```python
from build123d import *

# Parameters (mm, degrees)
SKETCH1_W           = 200
SKETCH1_H           = 35
BOSS_EXTRUDE1_DEPTH = 3
FILLET1_R           = 15
CUT_EXTRUDE1_DEPTH  = 102.564019219


with BuildPart() as part:
    # Sketch1 → Boss-Extrude1 (new body)
    with BuildSketch(Plane(origin=(0, 0, 0), x_dir=(1, 0, 0), z_dir=(0, 1, 0))):
        Rectangle(SKETCH1_W, SKETCH1_H)
    extrude(amount=BOSS_EXTRUDE1_DEPTH)

    # Fillet1
    fillet1_edges = [part.edges().sort_by_distance(p)[0] for p in [
        (100, 1.5, -17.5),
        (100, 1.5, 17.5),
    ]]
    fillet(fillet1_edges, radius=FILLET1_R)

    # Sketch2 → Cut-Extrude1 (cut, through all)
    with BuildSketch(Plane(origin=(0, 3, 0), x_dir=(1, 0, 0), z_dir=(0, 1, 0))):
        with BuildLine():
            ThreePointArc((-93.377001476, 15), (-96.147633262, 16.147633262), (-95, 13.377001476))
            Line((-95, 13.377001476), (-95, 15))
            Line((-95, 15), (-93.377001476, 15))
        make_face()
        with BuildLine():
            Line((-95, 15), (-95, 13.377001476))
            ThreePointArc((-95, 13.377001476), (-93.852366738, 13.852366738), (-93.377001476, 15))
            Line((-93.377001476, 15), (-95, 15))
        make_face()
        with BuildLine():
            ThreePointArc((-95, -13.5), (-96.060660172, -16.060660172), (-93.5, -15))
            Line((-93.5, -15), (-95, -15))
            Line((-95, -15), (-95, -13.5))
        make_face()
        with BuildLine():
            Line((-95, -15), (-93.5, -15))
            ThreePointArc((-93.5, -15), (-93.939339828, -13.939339828), (-95, -13.5))
            Line((-95, -13.5), (-95, -15))
        make_face()
        with BuildLine():
            ThreePointArc((-63.143993753, -13.5), (-64.204653925, -13.939339828), (-64.643993753, -15))
            Line((-64.643993753, -15), (-63.143993753, -15))
            Line((-63.143993753, -15), (-63.143993753, -13.5))
        make_face()
        with BuildLine():
            Line((-63.143993753, -15), (-64.643993753, -15))
            ThreePointArc((-64.643993753, -15), (-63.143993753, -16.5), (-61.643993753, -15))
            ThreePointArc((-61.643993753, -15), (-62.083333581, -13.939339828), (-63.143993753, -13.5))
            Line((-63.143993753, -13.5), (-63.143993753, -15))
        make_face()
        with BuildLine():
            ThreePointArc((-64.643993753, 15), (-64.204653925, 13.939339828), (-63.143993753, 13.5))
            Line((-63.143993753, 13.5), (-63.143993753, 15))
            Line((-63.143993753, 15), (-64.643993753, 15))
        make_face()
        with BuildLine():
            Line((-63.143993753, 15), (-63.143993753, 13.5))
            ThreePointArc((-63.143993753, 13.5), (-62.083333581, 13.939339828), (-61.643993753, 15))
            ThreePointArc((-61.643993753, 15), (-63.143993753, 16.5), (-64.643993753, 15))
            Line((-64.643993753, 15), (-63.143993753, 15))
        make_face()
    extrude(amount=-CUT_EXTRUDE1_DEPTH, mode=Mode.SUBTRACT)


solid = part.part
```
CAD build for the part. Positions are in the model's coordinates, mm. Give positions to 0.01 mm unless a question says otherwise; leave off trailing zeros. Write each loop counter-clockwise with the first axis right and the second up, starting at its lowest first coordinate (ties: lowest second). Pieces come first, ordered by that corner, then holes. Notation, with made-up numbers: M -25,-34 L -3,-34 A18 cw -3,-2 Z; hole C 41,-32 d10. An arc over 180 degrees is marked long. Return JSON: item names as keys, results as strings. Group by question number.
(1) Band-saw the part on A-A (y = 2.45). Give the cut face in (x, z), and give its area (3 significant figures).
(2) Drill centre lines: L1, parallel to Z at x = -95, y = 2.2; L2, parallel to X at y = 1.5, z = -15; L3, parallel to X at y = 2, z = 15. Where is each one in solid material? Low to high. Write a range as [from, to].
(3) Flat gauge pin, fed straight in: pin 1 Ø2.5 at (x, z) = (-95, -15) entering from -Y. Where does the tip first touch, or does it go through?
Entries:
{
 "1": {"outline": "M -100,-17.5 L 85,-17.5 A15 ccw 100,-2.5 L 100,2.5 A15 ccw 85,17.5 L -100,17.5 Z; hole C -95,-15 d3.25; hole C -95,15 d3; hole C -63.14,-15 d3; hole C -63.14,15 d3", "area": "6,870 mm^2"},
 "2": {"L1": "z = [-17.5, -16.62], [-13.38, 13.5], [16.5, 17.5]", "L2": "x = [-100, -96.62], [-93.38, -64.64], [-61.64, 93.29]", "L3": "x = [-100, -96.5], [-93.5, -64.64], [-61.64, 93.29]"},
 "3": {"pin 1": "passes through"}
}
